Answer from the drawing. Dimensions are ordinates in mm from the lowest x, y and z of the part. A direction names the side the tool comes from. Coordinates: 2 decimals unless noted, no trailing zeros. Order: outer loops, then holes, each group sorted by start corner. A loop starts at its lowest first (then second) coordinate and runs counter-clockwise, first axis right, second up. Notation, with made-up numbers: M -13.75,-40 L 33.25,-40 A26 ccw 33.25,-3 Z; hole C 37.5,-21 d8. An arc over 180 degrees is marked long. Use a Markdown table: item, result.
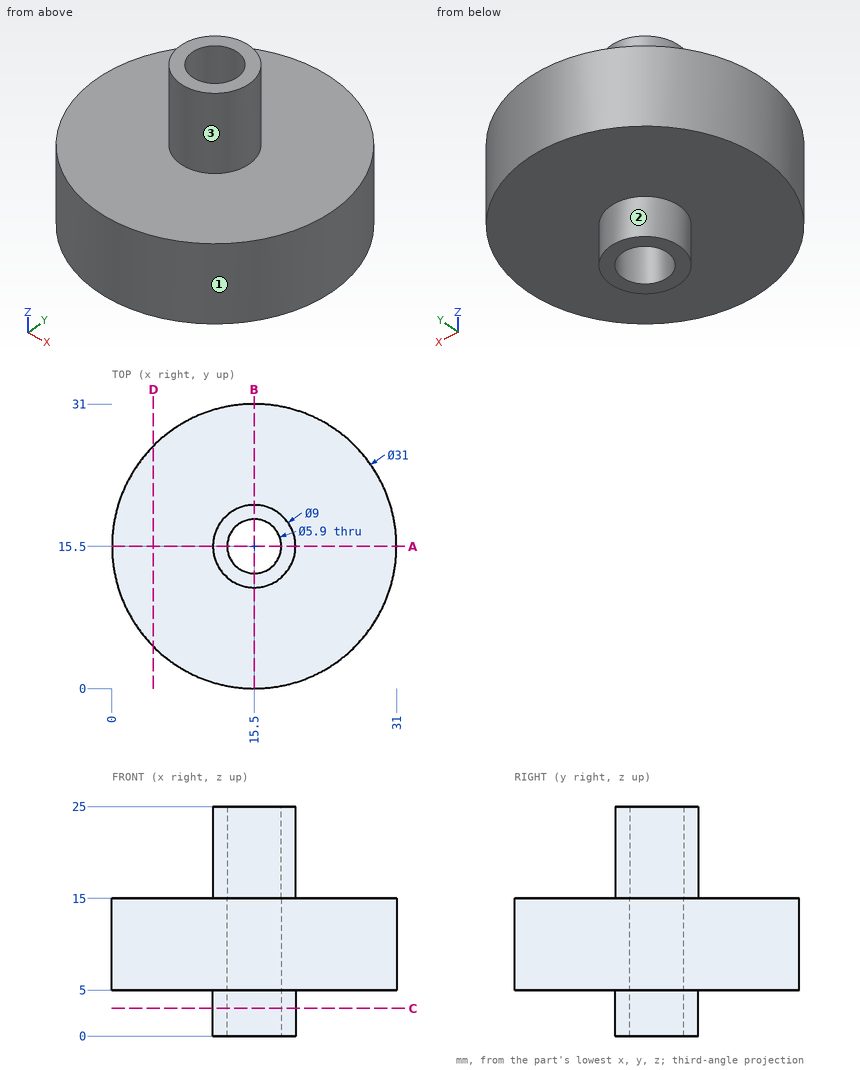
(1) A cutting plane is placed at C-C (z = 3). Determine the outline of the cut face in (x, y), then the cut area to 3 significant figures.
Conclusion:
| item | result |
|---|---|
| outline | C 15.5,15.5 d9; hole C 15.5,15.5 d5.9 |
| area | 36.3 mm2 |
(2) Straight lines are drawn through the part: L1, parallel to Y at x = 15.5, z = 8; L2, parallel to Z at x = 14, y = 28; L3, parallel to Y at x = 15.5, z = 21.25. For each, find the intervals that lie inside material, in ascending order.
Conclusion:
| item | result |
|---|---|
| L1 | 0 to 12.55, 18.45 to 31 |
| L2 | 5 to 15 |
| L3 | 11 to 12.55, 18.45 to 20 |
(3) A cutting plane is placed at D-D (x = 4.5). Determine the outline of the cut face in (y, z).
Conclusion:
| item | result |
|---|---|
| outline | M 4.58,5 L 26.42,5 L 26.42,15 L 4.58,15 Z |
(4) Which of the six approach directions +Z, -Z, +X, -X, +Y, -Y give full straight-line access (tool end or side, diameter ignored) to the marked faces 1, 2 and 3?
Conclusion:
| item | result |
|---|---|
| face 1 | +Z, -Z |
| face 2 | -Z |
| face 3 | +Z |
(5) Given P1, Ø2, axis at x = 16, z = 20, coming from the -Y side; P2, Ø1.5, axis at x = 8.5, z = 4, coming from the -Y side; P3, Ø4, axis at y = 24.5, z = 11.5, coming from the +X side; P4, Ø12, axis at x = 12, z = 8.5, coming from the -Y side, each flat-ended and moving along its own axis, determine where each tip first touches the part or whether it passes through.
Conclusion:
| item | result |
|---|---|
| P1 | y = 11 |
| P2 | through |
| P3 | x = 29.33 |
| P4 | y = 0 |
(6) A cutting plane is placed at A-A (y = 15.5). Determine the outline of the cut face in (x, z).
Conclusion:
| item | result |
|---|---|
| outline | M 0,5 L 11,5 L 11,0 L 12.55,0 L 12.55,25 L 11,25 L 11,15 L 0,15 Z; M 18.45,0 L 20,0 L 20,5 L 31,5 L 31,15 L 20,15 L 20,25 L 18.45,25 Z |
